Read the model definition and answer for the solid it produces. Units are mm, in the model's axes. Face numbers are marked on the shaded views. A direction names the side the tool comes from. Round coordinates to 2 decimals unless told otherwise and drop trailing zeros. Write each loop counter-clockwise with the first axis right and the second up, starting at its lowest first coordinate (ties: lowest second). Pieces come first, ordered by that corner, then holes. Notation, with made-up numbers: (35, 66) - (70, 66) arc R18 ccw to (70, 92) - close; hole circle Ø4 at (8.5, 79.5). An arc over 180 degrees is marked (long way). Use one line per item in the form item = value. Start each with the question number.
1) The part is cut by section C-C, the plane y = 7.75. Give the vertices of the cut face in (x, z), plus the area to 3 significant figures.
2) Each of these flat-tipped pins is pushed along its axis until it touches: pin 1 (4.5 mm diameter, centred on x = -0.5, y = 3.5, fed in from +Z); pin 2 (8 mm diameter, centred on x = -18.5, y = 15.5, fed in from +Z); pin 3 (6 mm diameter, centred on y = 6, z = 21.5, fed in from +X); pin 4 (7 mm diameter, centred on y = 10.12, z = 25.7, fed in from -X). Where does it stop, or does it pass through?
3) The part is cut by section D-D, the plane x = 5. Give the vertices of the cut face in (y, z), plus the area to 3 significant figures.
4) Consider line 1 along X through (y, z) = (9, 5); line 2 along Z through (x, y) = (31.5, 9.75); line 3 along X through (y, z) = (8.25, 17.5). Determine where each line is inside the solid, lowest interval first. Write a range as from..to.
5) The part is cut by section B-B, the plane z = 22. Give the vertices of the cut face in (x, y).
6) The part is cut by section A-A, the plane x = -21. Give the vertices of the cut face in (y, z), plus the area to 3 significant figures.
7) For a pull along X with two mould halves and no side action, classify the marked faces 4, 5 and 6 as released by +X, released by -X, zero draft, split by the parting line, or undercut.
8) For the marked faces 1, 2 and 3, determine the directions among +Z, -Z, +X, -X, +Y, -Y from which every point of the face is accessible in a straight line to the end or side of a thin tool.
Solid Edge part; units mm, degrees
sketch "Sketch1" plane through (0, 0, 0) normal (0, -1, 0) x (1, 0, 0)
  line L0 (-2.8327, 25.7018) -> (-2.8327, 7.8764)
  line L1 (-35.3055, 7.8764) -> (-2.8327, 7.8764)
  line L2 (-35.3055, 0) -> (-35.3055, 7.8764)
  line L3 (-30.3309, 0) -> (-35.3055, 0)
  line L4 (-30.3309, 0) -> (-30.3309, 3.9382)
  line L5 (-30.3309, 3.9382) -> (29.5018, 3.9382)
  line L6 (29.5018, 3.9382) -> (29.5018, 0)
  line L7 (36.5491, 0) -> (29.5018, 0)
  line L8 (36.5491, 7.8764) -> (36.5491, 0)
  line L9 (3.2473, 7.8764) -> (36.5491, 7.8764)
  line L10 (3.2473, 7.8764) -> (3.2473, 25.7018)
  line L11 (3.2473, 25.7018) -> (-2.8327, 25.7018)
extrude "Protrusion1" add sketch "Sketch1" against normal blind 20.2422
sketch "Sketch2" plane through (3.2473, 10.1211, 16.7891) normal (1, 0, 0) x (0, 1, 0)
  line L0 (-10.1211, 8.9127) -> (10.1211, 8.9127)
  arc A0 (-10.1211, 8.9127) -> (10.1211, 8.9127) centre (0, 8.9127) cw
extrude "ExtrudedProtrusion_2" add sketch "Sketch2" against normal blind 6
sketch "Sketch3" plane through (3.2473, 10.1211, 21.8496) normal (1, 0, 0) x (0, 1, 0)
  circle A0 centre (0, 3.8522) radius 4.4852
extrude "ExtrudedCutout_1" cut sketch "Sketch3" against normal blind 19.6871
hole "Hole_1" at (20.6248, 10.4844, 7.8764) direction (0, 0, -1) diameter 10 end up to next
hole "Hole1" at (-25.3309, 10.4844, 7.8764) direction (0, 0, -1) diameter 10 end up to next
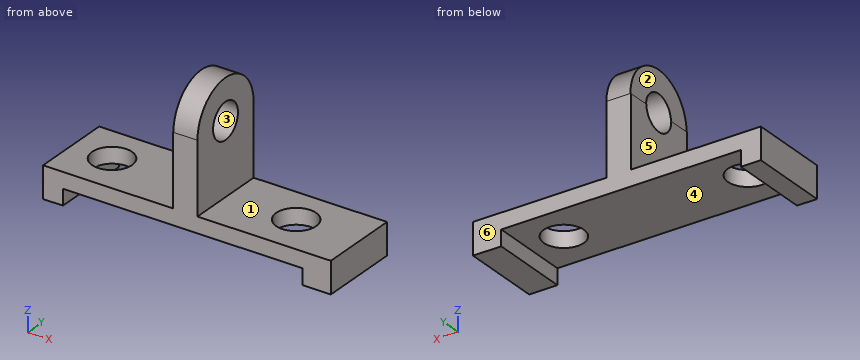
Geometry results:
q1.outline = (-35.31, 0) - (-30.33, 0) - (-30.33, 3.94) - (-29.52, 3.94) - (-29.52, 7.88) - (-35.31, 7.88) - close; (-21.14, 3.94) - (16.44, 3.94) - (16.44, 7.88) - (3.25, 7.88) - (3.25, 21.89) - (-2.83, 21.89) - (-2.83, 7.88) - (-21.14, 7.88) - close; (-2.75, 29.51) - (3.25, 29.51) - (3.25, 35.54) - (-2.75, 35.54) - close; (24.81, 3.94) - (29.5, 3.94) - (29.5, 0) - (36.55, 0) - (36.55, 7.88) - (24.81, 7.88) - close
q1.area = 386 mm2
q2.pin_1 = 34.83
q2.pin_2 = 7.88
q2.pin_3 = 3.25
q2.pin_4 = through
q3.outline = (0, 3.94) - (20.24, 3.94) - (20.24, 7.88) - (0, 7.88) - close
q3.area = 79.7 mm2
q4.line_1 = -35.31..-30.11, -20.56..15.85, 25.4..36.55
q4.line_2 = 0..7.88
q4.line_3 = -2.83..3.25
q5.outline = (-2.83, 0) - (3.25, 0) - (3.25, 7.59) - (-2.83, 7.59) - close; (-2.83, 12.65) - (3.25, 12.65) - (3.25, 20.24) - (-2.83, 20.24) - close
q6.outline = (0, 3.94) - (7.99, 3.94) - (7.99, 7.88) - (0, 7.88) - close; (12.98, 3.94) - (20.24, 3.94) - (20.24, 7.88) - (12.98, 7.88) - close
q6.area = 60.0 mm2
q7.face_4 = undercut
q7.face_5 = released by -X
q7.face_6 = zero draft
q8.face_1 = +Z, +X, +Y, -Y
q8.face_2 = +Z, -X, +Y, -Y
q8.face_3 = +X, -X
